Geometry check sheet. Reference: the model listing, model coordinates, mm. Give positions to 0.01 mm unless a question says otherwise; leave off trailing zeros. Loops run counter-clockwise (first coordinate to the right, second up) from the corner with the lowest first, then second, coordinate; pieces in that order, holes last. Notation, with made-up numbers: (38.5, 38.5) -> (81.5, 38.5) arc R7 cw to (81.5, 48.5) -> close; hole circle Ø9 at (6.5, 15). An arc over 180 degrees is marked (long way). Write item = value, one per line. Start each with the question number.
Autodesk Inventor part; units mm, degrees
ref_plane "YZ Plane" through (0, 0, 0) normal (1, 0, 0) x (0, 1, 0)
ref_plane "XZ Plane" through (0, 0, 0) normal (0, 1, 0) x (-1, 0, 0)
ref_plane "XY Plane" through (0, 0, 0) normal (0, 0, 1) x (1, 0, 0)
sketch "Absorber-Base" plane through (0, 0, 0) normal (0, 0, 1) x (1, 0, 0)
  line L0 (-20, 20) -> (20, 20)
  line L1 (20, 20) -> (20, -20)
  line L2 (20, -20) -> (-20, -20)
  line L3 (-20, -20) -> (-20, 20)
  line L4 (-20, 20) -> (20, -20) construction
  line L5 (20, 20) -> (-20, -20) construction
  point P0 (0, 0)
  dimension "d0" = 40
extrude "Gesamtvolumen" add sketch "Absorber-Base" along normal blind 60
sketch "Skizze2" plane through (0, 0, 0) normal (0, 1, 0) x (-1, 0, 0)
  line L0 (-28, 0) -> (28, 0)
  line L1 (20, 0) -> (20, 60)
  line L2 (-20, 0) -> (-20, 60)
  line L3 (20, 0) -> (-20, 0)
  line L4 (-20, 0) -> (-20, 10)
  line L5 (-20, 10) -> (20, 10)
  line L6 (20, 10) -> (20, 0)
  line L7 (-20, 60) -> (20, 60)
  line L8 (0, 60) -> (20, 10)
  line L9 (0, 60) -> (-20, 10)
  point P0 (0, 0)
  point P1 (20, 10)
  dimension "d6" = 10
extrude "Cutaway" cut sketch "Skizze2" along normal mid plane 40 contours L2 L7 L9 | L8 L7 L1
pattern_circular "Runde Anordnung1" count 2 over 90 about axis through (0, 0, -10) along (0, 0, 1) of "Cutaway"
equation "\"d0\" = Base_Seitenlänge"
equation "\"d1\" = Gesamthöhe"
equation "\"d6\" = Base_Höhe"
equation "\"d7\" = Base_Seitenlänge"
equation "\"Base_Seitenlänge\" = 40"
equation "\"Base_Höhe\" = 10"
equation "\"Gesamthöhe\" = 60"
properties part number "HF-Absorber-dummy"
1) Section check D-D (z = 39.5). Enter the section's corners in (x, y), plus the area to 3 significant figures.
2) Section check B-B (x = -10). Enter the section's corners in (y, z), plus the area to 3 significant figures.
3) Depth check by flat-ended pin: pin 1 Ø1.5 at (y, z) = (0.5, 31) entering from -X; pin 2 Ø10 at (y, z) = (-16, 38) entering from -X; pin 3 Ø1 at (y, z) = (-0.5, 37.5) entering from +X; pin 4 Ø12 at (x, z) = (8.5, 50) entering from -Y. Enter the tip coordinate at first touch or a pass-through.
4) Section check A-A (y = 12). Enter the section's corners in (x, z), plus the area to 3 significant figures.
5) Section check C-C (z = 22). Enter the section's corners in (x, y), plus the area to 3 significant figures.
6) Thickness scan on line 1 (Z direction, x = 1, y = -14); line 2 (Z direction, x = -13, y = 15.5); line 3 (X direction, y = 9.5, z = 22.5). Record the ranges inside material, lowest first.
Check result:
q1.outline = (-8.2, -8.2) -> (8.2, -8.2) -> (8.2, 8.2) -> (-8.2, 8.2) -> close
q1.area = 269 mm2
q2.outline = (-20, 0) -> (20, 0) -> (20, 10) -> (10, 35) -> (-10, 35) -> (-20, 10) -> close
q2.area = 1,150 mm2
q3.pin_1 = -11.9
q3.pin_2 = through
q3.pin_3 = 9.2
q3.pin_4 = -6.22
q4.outline = (-20, 0) -> (20, 0) -> (20, 10) -> (12, 30) -> (-12, 30) -> (-20, 10) -> close
q4.area = 1,040 mm2
q5.outline = (-15.2, -15.2) -> (15.2, -15.2) -> (15.2, 15.2) -> (-15.2, 15.2) -> close
q5.area = 924 mm2
q6.line_1 = 0 to 25
q6.line_2 = 0 to 21.25
q6.line_3 = -15 to 15
